from build123d import *

# Parameters (mm, degrees)
SKETCH4_R                  = 10
BOSS_EXTRUDE1_DEPTH        = 3.5
F_6_0MM_DOWEL_HOLE3_D      = 6
F_6_0MM_DOWEL_HOLE4_D      = 6
F_6_0MM_DOWEL_HOLE5_D      = 6
F_6_0MM_DOWEL_HOLE6_D      = 6
F_6_0MM_DOWEL_HOLE7_D      = 6
F_6_0MM_DOWEL_HOLE8_D      = 6
F_6_0MM_DOWEL_HOLE9_D      = 6
F_6_0MM_DOWEL_HOLE10_D     = 6
F_6_0MM_DOWEL_HOLE11_D     = 6
F_6_0MM_DOWEL_HOLE12_D     = 6
F_6_0MM_DOWEL_HOLE13_D     = 6
F_6_0MM_DOWEL_HOLE14_D     = 6
F_6_0MM_DOWEL_HOLE15_D     = 6
F_6_0MM_DOWEL_HOLE16_D     = 6
F_6_0MM_DOWEL_HOLE17_D     = 6
F_6_0MM_DOWEL_HOLE17_DEPTH = 30.64
F_6_0MM_DOWEL_HOLE17_TIP   = 1.802581857
F_6_0MM_DOWEL_HOLE18_D     = 6
F_6_0MM_DOWEL_HOLE18_DEPTH = 30.64
F_6_0MM_DOWEL_HOLE18_TIP   = 1.802581857
F_6_0MM_DOWEL_HOLE19_D     = 6
F_6_0MM_DOWEL_HOLE19_DEPTH = 30.64
F_6_0MM_DOWEL_HOLE19_TIP   = 1.802581857
F_6_0MM_DOWEL_HOLE20_D     = 6
F_6_0MM_DOWEL_HOLE20_DEPTH = 30.64
F_6_0MM_DOWEL_HOLE20_TIP   = 1.802581857
F_6_0MM_DOWEL_HOLE21_D     = 6
F_6_0MM_DOWEL_HOLE22_D     = 6
F_6_0MM_DOWEL_HOLE23_D     = 6
F_6_0MM_DOWEL_HOLE24_D     = 6
F_6_0MM_DOWEL_HOLE25_D     = 6
F_6_0MM_DOWEL_HOLE26_D     = 6
F_6_0MM_DOWEL_HOLE27_D     = 6
F_6_0MM_DOWEL_HOLE28_D     = 6
F_6_0MM_DOWEL_HOLE29_D     = 6
F_6_0MM_DOWEL_HOLE30_D     = 6


with BuildPart() as part:
    # Sketch4 → Boss-Extrude1 (new body)
    with BuildSketch(Plane(origin=(0, 0, 0), x_dir=(1, 0, 0), z_dir=(0, 1, 0))):
        Polygon((-36.7366, -50), (87.5, -50), (87.5, 0), (87.5, 130), (87.5, 170), (-36.7366, 98.239824704), (-36.7366, 58.239824704), (-36.7366, 23.58328615), align=None)
        with Locations(Location((67.5, 45.58328615, 0), (0, 0, 270))):
            Circle(SKETCH4_R, mode=Mode.SUBTRACT)
    extrude(amount=BOSS_EXTRUDE1_DEPTH)

    # Ø6.0mm Dowel Hole3 (through all)
    with Locations(Plane(origin=(-105.59791448, -96.5, 23.604755291), x_dir=(-1, 0, 0), z_dir=(0, -1, 0))):
        with Locations((-166.162017209, -5.414641336)):
            Hole(F_6_0MM_DOWEL_HOLE3_D / 2)

    # Ø6.0mm Dowel Hole4 (through all)
    with Locations(Plane(origin=(-105.59791448, 0, 23.604755291), x_dir=(-1, 0, 0), z_dir=(0, -1, 0))):
        with Locations((-166.162017209, -5.414641336)):
            Hole(F_6_0MM_DOWEL_HOLE4_D / 2)

    # Ø6.0mm Dowel Hole5 (through all)
    with Locations(Plane(origin=(-105.59791448, -96.5, 23.604755291), x_dir=(-1, 0, 0), z_dir=(0, -1, 0))):
        with Locations((-166.175485163, 27.545698678)):
            Hole(F_6_0MM_DOWEL_HOLE5_D / 2)

    # Ø6.0mm Dowel Hole6 (through all)
    with Locations(Plane(origin=(-105.59791448, 0, 23.604755291), x_dir=(-1, 0, 0), z_dir=(0, -1, 0))):
        with Locations((-166.175485163, 27.545698678)):
            Hole(F_6_0MM_DOWEL_HOLE6_D / 2)

    # Ø6.0mm Dowel Hole7 (through all)
    with Locations(Plane(origin=(-105.59791448, -96.5, 23.604755291), x_dir=(-1, 0, 0), z_dir=(0, -1, 0))):
        with Locations((-95.797211751, 27.547482752)):
            Hole(F_6_0MM_DOWEL_HOLE7_D / 2)

    # Ø6.0mm Dowel Hole8 (through all)
    with Locations(Plane(origin=(-105.59791448, 0, 23.604755291), x_dir=(-1, 0, 0), z_dir=(0, -1, 0))):
        with Locations((-95.797211751, 27.547482752)):
            Hole(F_6_0MM_DOWEL_HOLE8_D / 2)

    # Ø6.0mm Dowel Hole9 (through all)
    with Locations(Plane(origin=(-105.59791448, -96.5, 23.604755291), x_dir=(-1, 0, 0), z_dir=(0, -1, 0))):
        with Locations((-83.36131448, 100.914726135)):
            Hole(F_6_0MM_DOWEL_HOLE9_D / 2)

    # Ø6.0mm Dowel Hole10 (through all)
    with Locations(Plane(origin=(-105.59791448, 0, 23.604755291), x_dir=(-1, 0, 0), z_dir=(0, -1, 0))):
        with Locations((-83.36131448, 100.914726135)):
            Hole(F_6_0MM_DOWEL_HOLE10_D / 2)

    # Ø6.0mm Dowel Hole11 (through all)
    with Locations(Plane(origin=(-105.59791448, -96.5, 23.604755291), x_dir=(-1, 0, 0), z_dir=(0, -1, 0))):
        with Locations((-116.36131448, 100.914726135)):
            Hole(F_6_0MM_DOWEL_HOLE11_D / 2)

    # Ø6.0mm Dowel Hole12 (through all)
    with Locations(Plane(origin=(-105.59791448, 0, 23.604755291), x_dir=(-1, 0, 0), z_dir=(0, -1, 0))):
        with Locations((-116.36131448, 100.914726135)):
            Hole(F_6_0MM_DOWEL_HOLE12_D / 2)

    # Ø6.0mm Dowel Hole13 (through all)
    with Locations(Plane(origin=(-105.59791448, -96.5, 23.604755291), x_dir=(-1, 0, 0), z_dir=(0, -1, 0))):
        with Locations((-116.36131448, 68.191325462)):
            Hole(F_6_0MM_DOWEL_HOLE13_D / 2)

    # Ø6.0mm Dowel Hole14 (through all)
    with Locations(Plane(origin=(-105.59791448, 0, 23.604755291), x_dir=(-1, 0, 0), z_dir=(0, -1, 0))):
        with Locations((-116.36131448, 68.191325462)):
            Hole(F_6_0MM_DOWEL_HOLE14_D / 2)

    # Ø6.0mm Dowel Hole15 (through all)
    with Locations(Plane(origin=(-105.59791448, -96.5, 23.604755291), x_dir=(-1, 0, 0), z_dir=(0, -1, 0))):
        with Locations((-83.401438286, 68.177816696)):
            Hole(F_6_0MM_DOWEL_HOLE15_D / 2)

    # Ø6.0mm Dowel Hole16 (through all)
    with Locations(Plane(origin=(-105.59791448, 0, 23.604755291), x_dir=(-1, 0, 0), z_dir=(0, -1, 0))):
        with Locations((-83.401438286, 68.177816696)):
            Hole(F_6_0MM_DOWEL_HOLE16_D / 2)

    # Ø6.0mm Dowel Hole17
    with Locations(Plane(origin=(-105.59791448, 3.5, 23.604755291), x_dir=(1, 0, 0), z_dir=(0, 1, 0))):
        with Locations((83.614280544, 84.439845005)):
            Hole(F_6_0MM_DOWEL_HOLE17_D / 2, depth=F_6_0MM_DOWEL_HOLE17_DEPTH)
            with Locations((0, 0, -(F_6_0MM_DOWEL_HOLE17_DEPTH + F_6_0MM_DOWEL_HOLE17_TIP / 2))):  # 118° drill point
                Cone(0, F_6_0MM_DOWEL_HOLE17_D / 2, F_6_0MM_DOWEL_HOLE17_TIP, mode=Mode.SUBTRACT)

    # Ø6.0mm Dowel Hole18
    with Locations(Plane(origin=(-105.59791448, 3.5, 23.604755291), x_dir=(1, 0, 0), z_dir=(0, 1, 0))):
        with Locations((116.294424018, 84.527773094)):
            Hole(F_6_0MM_DOWEL_HOLE18_D / 2, depth=F_6_0MM_DOWEL_HOLE18_DEPTH)
            with Locations((0, 0, -(F_6_0MM_DOWEL_HOLE18_DEPTH + F_6_0MM_DOWEL_HOLE18_TIP / 2))):  # 118° drill point
                Cone(0, F_6_0MM_DOWEL_HOLE18_D / 2, F_6_0MM_DOWEL_HOLE18_TIP, mode=Mode.SUBTRACT)

    # Ø6.0mm Dowel Hole19
    with Locations(Plane(origin=(-105.59791448, 3.5, 23.604755291), x_dir=(1, 0, 0), z_dir=(0, 1, 0))):
        with Locations((99.602293645, 67.882806011)):
            Hole(F_6_0MM_DOWEL_HOLE19_D / 2, depth=F_6_0MM_DOWEL_HOLE19_DEPTH)
            with Locations((0, 0, -(F_6_0MM_DOWEL_HOLE19_DEPTH + F_6_0MM_DOWEL_HOLE19_TIP / 2))):  # 118° drill point
                Cone(0, F_6_0MM_DOWEL_HOLE19_D / 2, F_6_0MM_DOWEL_HOLE19_TIP, mode=Mode.SUBTRACT)

    # Ø6.0mm Dowel Hole20
    with Locations(Plane(origin=(-105.59791448, 3.5, 23.604755291), x_dir=(1, 0, 0), z_dir=(0, 1, 0))):
        with Locations((99.658582024, 100.737664948)):
            Hole(F_6_0MM_DOWEL_HOLE20_D / 2, depth=F_6_0MM_DOWEL_HOLE20_DEPTH)
            with Locations((0, 0, -(F_6_0MM_DOWEL_HOLE20_DEPTH + F_6_0MM_DOWEL_HOLE20_TIP / 2))):  # 118° drill point
                Cone(0, F_6_0MM_DOWEL_HOLE20_D / 2, F_6_0MM_DOWEL_HOLE20_TIP, mode=Mode.SUBTRACT)

    # Ø6.0mm Dowel Hole21 (through all)
    with Locations(Plane(origin=(-105.59791448, -96.5, 23.604755291), x_dir=(-1, 0, 0), z_dir=(0, -1, 0))):
        with Locations((-173.858224897, 126.122531585)):
            Hole(F_6_0MM_DOWEL_HOLE21_D / 2)

    # Ø6.0mm Dowel Hole22 (through all)
    with Locations(Plane(origin=(-105.59791448, 0, 23.604755291), x_dir=(-1, 0, 0), z_dir=(0, -1, 0))):
        with Locations((-173.858224897, 126.122531585)):
            Hole(F_6_0MM_DOWEL_HOLE22_D / 2)

    # Ø6.0mm Dowel Hole23 (through all)
    with Locations(Plane(origin=(-105.59791448, -96.5, 23.604755291), x_dir=(-1, 0, 0), z_dir=(0, -1, 0))):
        with Locations((-157.37079531, 154.603853756)):
            Hole(F_6_0MM_DOWEL_HOLE23_D / 2)

    # Ø6.0mm Dowel Hole24 (through all)
    with Locations(Plane(origin=(-105.59791448, 0, 23.604755291), x_dir=(-1, 0, 0), z_dir=(0, -1, 0))):
        with Locations((-157.37079531, 154.603853756)):
            Hole(F_6_0MM_DOWEL_HOLE24_D / 2)

    # Ø6.0mm Dowel Hole25 (through all)
    with Locations(Plane(origin=(-105.59791448, -96.5, 23.604755291), x_dir=(-1, 0, 0), z_dir=(0, -1, 0))):
        with Locations((-124.287288406, 135.474563451)):
            Hole(F_6_0MM_DOWEL_HOLE25_D / 2)

    # Ø6.0mm Dowel Hole26 (through all)
    with Locations(Plane(origin=(-105.59791448, 0, 23.604755291), x_dir=(-1, 0, 0), z_dir=(0, -1, 0))):
        with Locations((-124.287288406, 135.474563451)):
            Hole(F_6_0MM_DOWEL_HOLE26_D / 2)

    # Ø6.0mm Dowel Hole27 (through all)
    with Locations(Plane(origin=(-105.59791448, -96.5, 23.604755291), x_dir=(-1, 0, 0), z_dir=(0, -1, 0))):
        with Locations((-140.764255961, 106.890061518)):
            Hole(F_6_0MM_DOWEL_HOLE27_D / 2)

    # Ø6.0mm Dowel Hole28 (through all)
    with Locations(Plane(origin=(-105.59791448, 0, 23.604755291), x_dir=(-1, 0, 0), z_dir=(0, -1, 0))):
        with Locations((-140.764255961, 106.890061518)):
            Hole(F_6_0MM_DOWEL_HOLE28_D / 2)

    # Ø6.0mm Dowel Hole29 (through all)
    with Locations(Plane(origin=(-105.59791448, -96.5, 23.604755291), x_dir=(-1, 0, 0), z_dir=(0, -1, 0))):
        with Locations((-95.797211751, -5.414641336)):
            Hole(F_6_0MM_DOWEL_HOLE29_D / 2)

    # Ø6.0mm Dowel Hole30 (through all)
    with Locations(Plane(origin=(-105.59791448, 0, 23.604755291), x_dir=(-1, 0, 0), z_dir=(0, -1, 0))):
        with Locations((-95.797211751, -5.414641336)):
            Hole(F_6_0MM_DOWEL_HOLE30_D / 2)


solid = part.part
Here's how the part is built. I have some questions about the finished solid (model axes, mm). Give positions to 0.01 mm unless a question says otherwise; leave off trailing zeros. Order: outer loops, then holes, each group sorted by start corner. A loop starts at its lowest first (then second) coordinate and runs counter-clockwise, first axis right, second up. Notation, with made-up numbers: (-23, 85) -> (4, 85) arc R27 ccw to (4, 106) -> close; hole circle Ø8 at (-11, -21). An arc over 180 degrees is marked (long way). Use a Markdown table: item, result. Add a question column.
Item 1: Imagine slicing it at D-D on x = 24. Please give me the cut outline in (y, z), plus the area to 3 significant figures.
Item 2: Will this pin go through, and if not, where does the flat tip stop? pin 1 (2 mm diameter, centred on x = 35, y = 2, fed in from -Z).
Item 3: I need wall thicknesses on line 1 (Z direction, x = 71, y = 0.4); line 2 (Z direction, x = -10, y = 2.85); line 3 (Z direction, x = 62.5, y = 0.85). Which ranges of each line are inside material? Lowest first, please.
Item 4: Imagine slicing it at C-C on y = 2.4. Give the number of separate pieces and of enclosed holes in the cut face, plus the area to 3 significant figures.
Item 5: Imagine slicing it at B-B on x = 67.5. Please give me the cut outline in (y, z).
Item 6: Imagine slicing it at A-A on z = -52. Please give me the cut outline in (x, y).
Item 7: If we mould it in two halves opening along X, with no side actions, what happens to faces 1 (the face through (25, 0, -37)), 2 (the face through (-8.8, 1.73, -78.03)), 3 (the face through (26.25, 1.73, -134.62))? For each: pulls with the +X half, pulls with the -X half, needs draft (parallel to the pull), parting line crosses it, or undercut.
Data:
| question | item | result |
|---|---|---|
| 1 | outline | (0, -133.32) -> (3.5, -133.32) -> (3.5, 50) -> (0, 50) -> close |
| 1 | area | 642 mm² |
| 2 | pin 1 | stops at z = -140.25 |
| 3 | line 1 | z = -160.47 to -103.74, -101.3 to -54.95, -36.22 to 50 |
| 3 | line 2 | z = -113.68 to -6.94, -0.95 to 26.03, 32.01 to 50 |
| 3 | line 3 | z = -155.56 to -54.24, -36.92 to -6.24, -1.64 to 26.73, 31.31 to 50 |
| 4 | separate pieces | 1 |
| 4 | enclosed holes | 17 |
| 4 | area | 22,100 mm² |
| 5 | outline | (0, -158.45) -> (3.5, -158.45) -> (3.5, -105.42) -> (0, -105.42) -> close; (0, -99.62) -> (3.5, -99.62) -> (3.5, -55.58) -> (0, -55.58) -> close; (0, -35.58) -> (3.5, -35.58) -> (3.5, 50) -> (0, 50) -> close |
| 6 | outline | (-36.74, 0) -> (59.83, 0) -> (59.83, 3.5) -> (-36.74, 3.5) -> close; (75.17, 0) -> (87.5, 0) -> (87.5, 3.5) -> (75.17, 3.5) -> close |
| 7 | face 1 | needs draft |
| 7 | face 2 | undercut |
| 7 | face 3 | pulls with the -X half |
